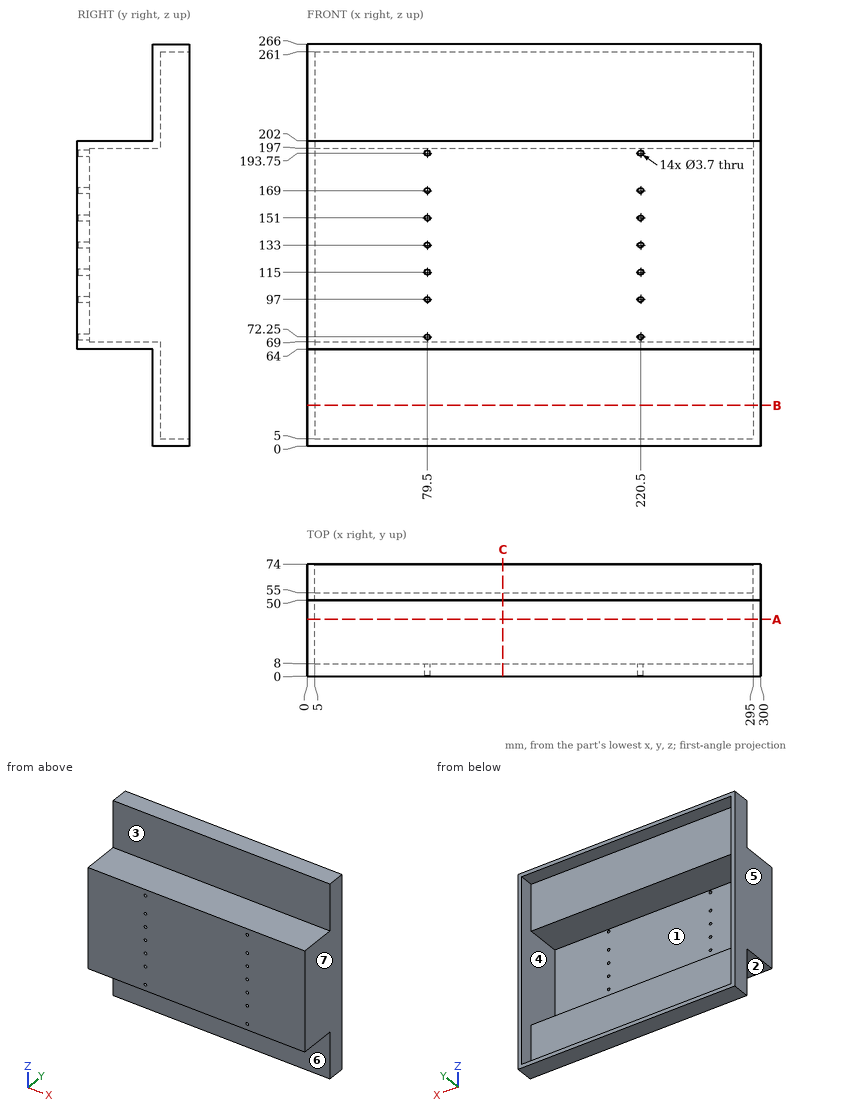
Verification items for this drawing (mm, ordinates from the low corner). A direction names the side the tool comes from. Coordinates: 2 decimals unless noted, no trailing zeros. Write each loop counter-clockwise with the first axis right and the second up, starting at its lowest first coordinate (ties: lowest second). Pieces come first, ordered by that corner, then holes. Notation, with made-up numbers: M 27,-7 L 83,-7 A24 ccw 83,5 Z; hole C 55.5,51 d3. An arc over 180 degrees is marked long. One line per item, written item: value. Start each with the question number.
(1) Sectioned sample at A-A, the plane y = 37.5. Enter the section's corners in (x, z).
(2) Scan lines: line 1 along X through (y, z) = (5.75, 97); line 2 along Z through (x, y) = (72, 56.5); line 3 along Z through (x, y) = (154, 8.5). Record each from-to range of solid material in increasing order. Write a range as [from, to].
(3) Tool access check on the marked faces 1, 2 and 3. Record the directions out of +Z, -Z, +X, -X, +Y, -Y that give a thin tool (end or side, any length) a straight path to the whole face; none if there is none.
(4) Depth check by flat-ended pin: pin 1 (4 mm diameter, centred on x = 175, z = 37, fed in from +Y); pin 2 (3.5 mm diameter, centred on x = 220.5, z = 151, fed in from -Y); pin 3 (1 mm diameter, centred on x = 193, y = 10, fed in from +Z); pin 4 (6 mm diameter, centred on x = 79.5, z = 115, fed in from +Y). Enter the tip coordinate at first touch or a pass-through.
(5) Sectioned sample at C-C, the plane x = 129.5. Enter the section's corners in (y, z), and give its area (3 significant figures).
(6) Release check for a two-part mould opening along X. For the marked faces 4, 5, 6 and 7 record: released by +X, released by -X, zero draft, split by the parting line, or undercut.
(7) Sectioned sample at B-B, the plane z = 27. Enter the section's corners in (x, y), and give its area (3 significant figures).
Filled sheet:
1. outline: M 0,64 L 300,64 L 300,202 L 0,202 Z; hole M 5,69 L 295,69 L 295,197 L 5,197 Z
2. line 1: [0, 77.65], [81.35, 218.65], [222.35, 300]
2. line 2: [0, 5], [261, 266]
2. line 3: [64, 69], [197, 202]
3. face 1: +Y
3. face 2: -Z, +X, -X, -Y
3. face 3: +Z, +X, -X, -Y
4. pin 1: y = 55
4. pin 2: through
4. pin 3: z = 202
4. pin 4: y = 8
5. outline: M 0,64 L 50,64 L 50,0 L 74,0 L 74,5 L 55,5 L 55,69 L 8,69 L 8,197 L 55,197 L 55,261 L 74,261 L 74,266 L 50,266 L 50,202 L 0,202 Z
5. area: 2,400 mm²
6. face 4: undercut
6. face 5: released by -X
6. face 6: zero draft
6. face 7: released by +X
7. outline: M 0,50 L 300,50 L 300,74 L 295,74 L 295,55 L 5,55 L 5,74 L 0,74 Z
7. area: 1,690 mm²
